from build123d import *

# Parameters (mm, degrees)
SKETCH_1_W          = 17
SKETCH_1_H          = 6.5
EXTRUDE_1_DEPTH     = 22.5
SKETCH_2_W          = 7
SKETCH_2_H          = 3.3
CUT_EXTRUDE_1_DEPTH = 23.5
SKETCH_3_R          = 1.15
CUT_EXTRUDE_2_DEPTH = 4


with BuildPart() as part:
    # 草图1 → 凸台-拉伸1 (new body)
    with BuildSketch(Plane.XY):
        Rectangle(SKETCH_1_W, SKETCH_1_H)
    extrude(amount=EXTRUDE_1_DEPTH)

    # 草图2 → 切除-拉伸1 (cut, through all)
    with BuildSketch(Plane.XY.offset(22.5)):
        with Locations((0, -1.6)):
            Rectangle(SKETCH_2_W, SKETCH_2_H)
    extrude(amount=-CUT_EXTRUDE_1_DEPTH, mode=Mode.SUBTRACT)

    # 草图3 → 切除-拉伸2 (cut)
    with BuildSketch(Plane(origin=(0, 3.25, 0), x_dir=(1, 0, 0), z_dir=(0, 1, 0))):
        with Locations((-6, -7.25)):
            Circle(SKETCH_3_R)
        with Locations((-6, -15.25)):
            Circle(SKETCH_3_R)
        with Locations((6, -15.25)):
            Circle(SKETCH_3_R)
        with Locations((6, -7.25)):
            Circle(SKETCH_3_R)
    extrude(amount=-CUT_EXTRUDE_2_DEPTH, mode=Mode.SUBTRACT)


solid = part.part
CAD build for the part. Positions are in the model's coordinates, mm. A direction names the side the tool comes from. Coordinates: 2 decimals unless noted, no trailing zeros. Loops run counter-clockwise (first coordinate to the right, second up) from the corner with the lowest first, then second, coordinate; pieces in that order, holes last. Notation, with made-up numbers: (-29.5, -24) - (-8.5, -24) arc R5 cw to (-8.5, -16) - close; hole circle Ø3 at (47.25, 79.5). An arc over 180 degrees is marked (long way). Write item = value, one per line. Start each with the question number.
Q1. Cut at B-B, the plane y = -1.25. List the corners of the cut face in (x, z).
Q2. Which spindle directions (+Z, -Z, +X, -X, +Y, -Y) get a long thin tool onto all of the face, cutting with end or side? Do faces 1 (the cylindrical face through (4.85, 1.28, 15.2)), 2 (the flat face through (-3.5, -2, 11)), 3 (the flat face through (6, -3.25, 11)). Say none if no direction does.
Q3. Cut at C-C, the plane z = 7.25. List the corners of the cut face in (x, y), then the cut area to 3 significant figures.
Q4. Cut at A-A, the plane y = 1.75. List the corners of the cut face in (x, z), then the cut area to 3 significant figures.
Q5. Pull direction X, two halves, no side cores. Call faces 4 (the flat face through (6, -0.75, 7)), 5 (the flat face through (-8.5, 0, 11)), 6 (the flat face through (0, 1, 22.5)): pulls with the +X half, pulls with the -X half, needs draft (parallel to the pull), parting line crosses it, or undercut.
Q6. Drill centre lines: L1, parallel to Z at x = -6, y = 1.9; L2, parallel to X at y = 0.65, z = 15.25; L3, parallel to X at y = -1.5, z = 21.25. Where is each one in solid material? Low to high.
Q7. Flat gauge pins, fed straight in: pin 1 Ø0.7 at (x, z) = (-6.5, 7) entering from +Y; pin 2 Ø3.5 at (x, z) = (1, 13) entering from -Y. Where does each tip first touch, or does it go through?
Q8. Cut at D-D, the plane x = 6. List the corners of the cut face in (y, z), then the cut area to 3 significant figures.
Computed:
q1.outline = (-8.5, 0) - (-3.5, 0) - (-3.5, 22.5) - (-8.5, 22.5) - close; (3.5, 0) - (8.5, 0) - (8.5, 22.5) - (3.5, 22.5) - close
q2.face_1 = +Y
q2.face_2 = +Z, -Z, -Y
q2.face_3 = +Z, -Z, +X, -X, -Y
q3.outline = (-8.5, -3.25) - (-3.5, -3.25) - (-3.5, 0.05) - (3.5, 0.05) - (3.5, -3.25) - (8.5, -3.25) - (8.5, 3.25) - (7.15, 3.25) - (7.15, -0.75) - (4.85, -0.75) - (4.85, 3.25) - (-4.85, 3.25) - (-4.85, -0.75) - (-7.15, -0.75) - (-7.15, 3.25) - (-8.5, 3.25) - close
q3.area = 69.0 mm²
q4.outline = (-8.5, 0) - (8.5, 0) - (8.5, 22.5) - (-8.5, 22.5) - close; hole circle Ø2.3 at (-6, 7.25); hole circle Ø2.3 at (-6, 15.25); hole circle Ø2.3 at (6, 7.25); hole circle Ø2.3 at (6, 15.25)
q4.area = 366 mm²
q5.face_4 = undercut
q5.face_5 = pulls with the -X half
q5.face_6 = needs draft
q6.L1 = 0 to 6.1, 8.4 to 14.1, 16.4 to 22.5
q6.L2 = -8.5 to -7.15, -4.85 to 4.85, 7.15 to 8.5
q6.L3 = -8.5 to -3.5, 3.5 to 8.5
q7.pin_1 = -0.75
q7.pin_2 = 0.05
q8.outline = (-3.25, 0) - (3.25, 0) - (3.25, 6.1) - (-0.75, 6.1) - (-0.75, 8.4) - (3.25, 8.4) - (3.25, 14.1) - (-0.75, 14.1) - (-0.75, 16.4) - (3.25, 16.4) - (3.25, 22.5) - (-3.25, 22.5) - close
q8.area = 128 mm²
